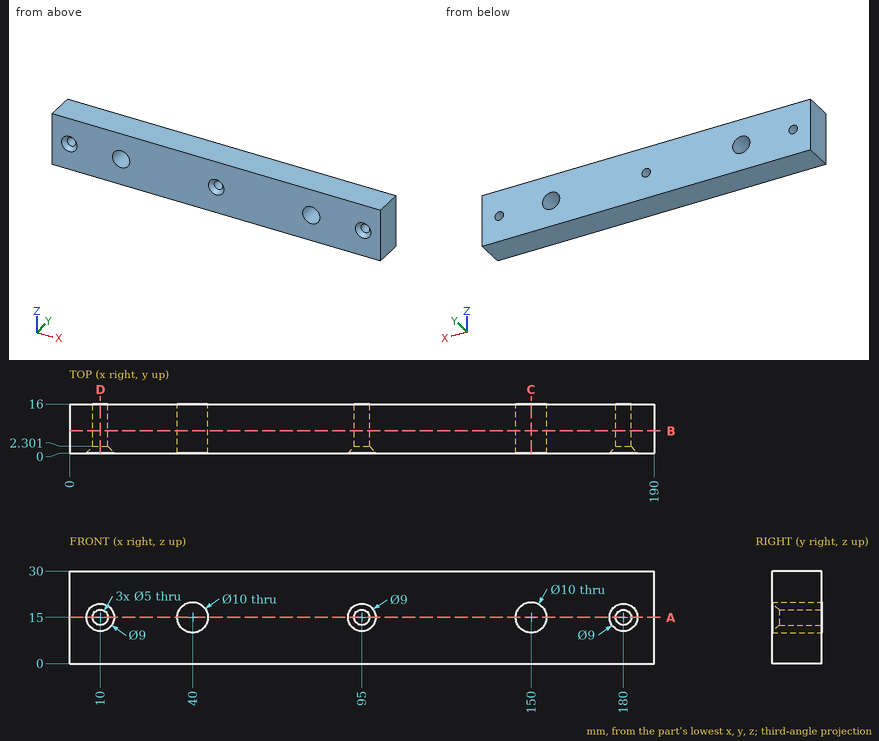
Answer from the drawing. Dimensions are ordinates in mm from the lowest x, y and z of the part. Give positions to 0.01 mm unless a question says otherwise; leave off trailing zeros. Loops run counter-clockwise (first coordinate to the right, second up) from the corner with the lowest first, then second, coordinate; pieces in that order, holes last.
Item 1: The part is cut by section B-B (y = 7.25). Write down the section's boundary in (x, z), and give its area (3 significant figures).
Item 2: The part is cut by section D-D (x = 10). Write down the section's boundary in (y, z), and give its area (3 significant figures).
Item 3: Each of these flat-tipped pins is pushed along its axis until it touches: pin 1 Ø8 at (x, z) = (180, 15) entering from +Y; pin 2 Ø8 at (x, z) = (40, 15) entering from +Y; pin 3 Ø8 at (x, z) = (10, 15) entering from -Y (1 decimal). Where does it stop, or does it pass through?
Item 4: The part is cut by section C-C (x = 150). Write down the section's boundary in (y, z), and give its area (3 significant figures).
Item 5: Find the intervals of material crossed by line 1 along Z through (x, y) = (10, 6.75); line 2 along Z through (x, y) = (150, 12); line 3 along X through (y, z) = (4, 14), in increasing order.
Item 6: The part is cut by section A-A (z = 15). Give the number of separate pieces and of enclosed holes in the cut face, and give its area (3 significant figures).
Taken from the geometry:
1. outline: (0, 0) - (190, 0) - (190, 30) - (0, 30) - close; hole circle Ø5 at (10, 15); hole circle Ø10 at (40, 15); hole circle Ø5 at (95, 15); hole circle Ø10 at (150, 15); hole circle Ø5 at (180, 15)
1. area: 5,480 mm2
2. outline: (0, 0) - (16, 0) - (16, 12.5) - (2.3, 12.5) - (0, 10.5) - close; (0, 19.5) - (2.3, 17.5) - (16, 17.5) - (16, 30) - (0, 30) - close
2. area: 395 mm2
3. pin 1: stops at y = 16
3. pin 2: passes through
3. pin 3: stops at y = 0.6
4. outline: (0, 0) - (16, 0) - (16, 10) - (0, 10) - close; (0, 20) - (16, 20) - (16, 30) - (0, 30) - close
4. area: 320 mm2
5. line 1: z = 0 to 12.5, 17.5 to 30
5. line 2: z = 0 to 10, 20 to 30
5. line 3: x = 0 to 7.71, 12.29 to 35.1, 44.9 to 92.71, 97.29 to 145.1, 154.9 to 177.71, 182.29 to 190
6. separate pieces: 6
6. enclosed holes: 0
6. area: 2,470 mm2
